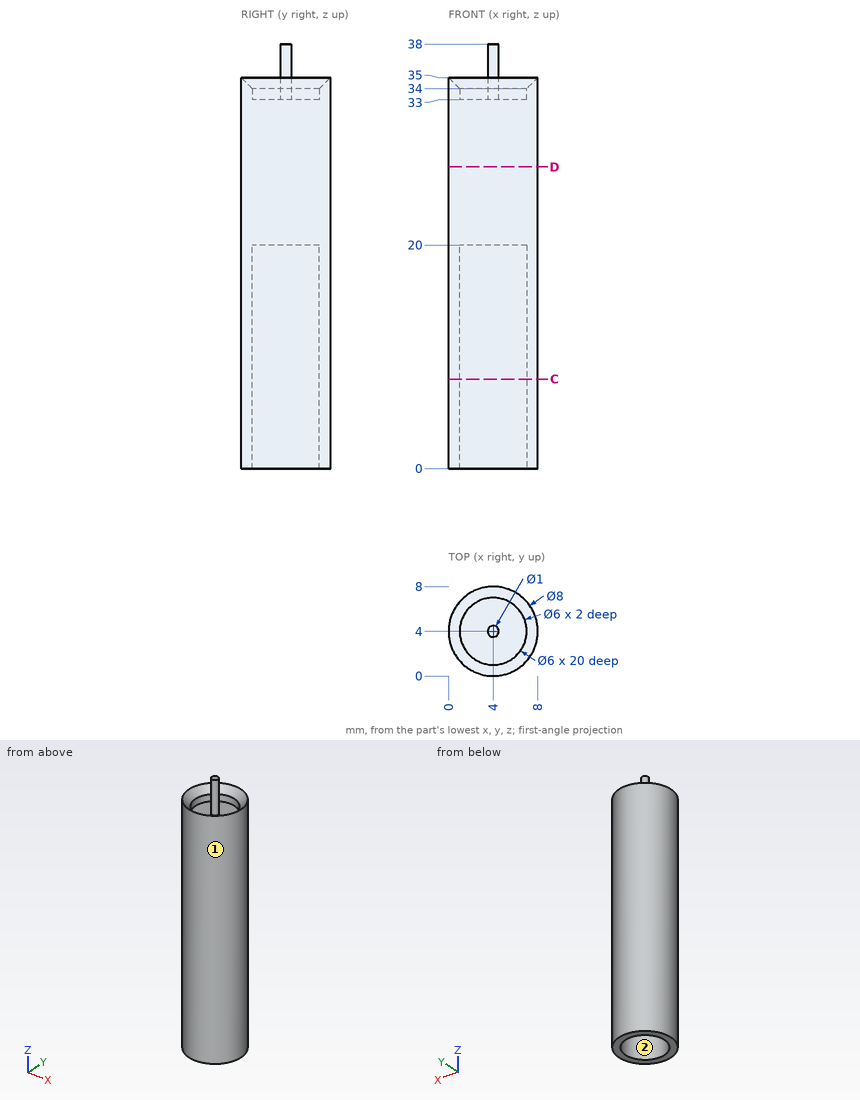
Geometry: see drawing. Coordinates: mm, zero at the bounding-box minimum. Coordinates: 2 decimals unless noted, no trailing zeros. Order: outer loops, then holes, each group sorted by start corner. A loop starts at its lowest first (then second) coordinate and runs counter-clockwise, first axis right, second up. Notation, with made-up numbers: (44.5, -28.75) - (87.5, -28.75) arc R6 cw to (87.5, -22.75) - close; hole circle Ø4 at (12, 83.25). An arc over 180 degrees is marked (long way). Return JSON: item names as keys, results as strings.
Q1. First-contact query: pin 1 (1 mm diameter, centred on x = 1.5, z = 13, fed in from -Y); pin 2 (1 mm diameter, centred on y = 1, z = 31, fed in from +X); pin 3 (2 mm diameter, centred on y = 1.5, z = 17.5, fed in from +X). Flat tips, straight axial feed; report the tip coordinate or a pass-through.
The answers:
{"pin 1": "stops at y = 0.54", "pin 2": "stops at x = 7.12", "pin 3": "stops at x = 7.71"}
Q2. Cut plane C-C (z = 8). Return loops of the section in (x, y), then the cut area to 3 significant figures.
The answers:
{"outline": "circle Ø8 at (4, 4); hole circle Ø6 at (4, 4)", "area": "22.0 mm2"}
Q3. Draft query along Y for the marked faces 1 and 2. Return one class per face: +Y half, -Y half, draft (parallel to the pull), parting line (faces both ways), or undercut.
The answers:
{"face 1": "parting line", "face 2": "undercut"}
Q4. Ray query, probe 1 along Y at (x, z) = (4, 33.3); probe 2 along Y at (x, z) = (4, 13.75); probe 3 along Y at (x, z) = (6.5, 10.5). Return the intervals inside material, ascending.
The answers:
{"probe 1": "y = 0 to 1, 3.5 to 4.5, 7 to 8", "probe 2": "y = 0 to 1, 7 to 8", "probe 3": "y = 0.88 to 2.34, 5.66 to 7.12"}
Q5. Cut plane D-D (z = 27). Return loops of the section in (x, y), then the cut area to 3 significant figures.
The answers:
{"outline": "circle Ø8 at (4, 4)", "area": "50.3 mm2"}
